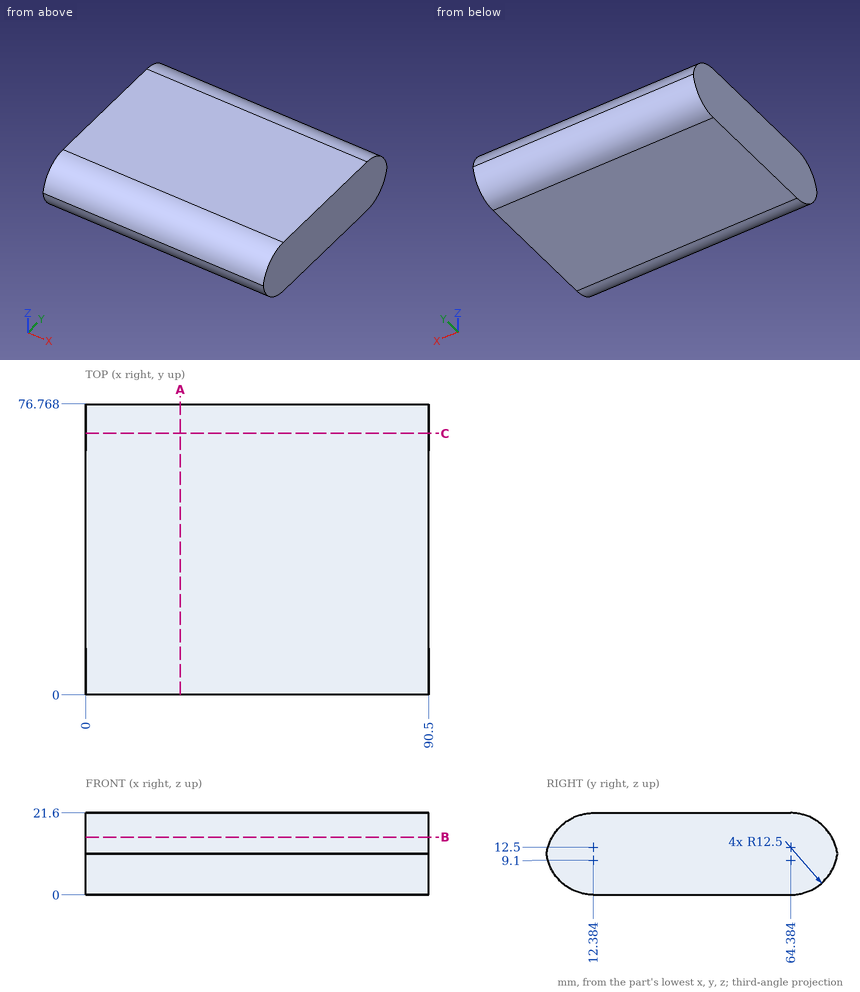
For this review, use the dimensioned drawing (mm, ordinates from the lowest corner) and the shaded views. Give positions to 0.01 mm unless a question says otherwise; leave off trailing zeros. Order: outer loops, then holes, each group sorted by start corner. A loop starts at its lowest first (then second) coordinate and runs counter-clockwise, first axis right, second up.
1) Take a section at C-C (y = 69). Give the boundary of the cut face in (x, z), then the cut area to 4 significant figures.
2) Take a section at A-A (x = 25). Give the boundary of the cut face in (y, z).
3) Wall thickness on line 1 (Z direction, x = 9, y = 65) (1 decimal); line 2 (Z direction, x = 36, y = 6); line 3 (Y direction, x = 17, z = 20) (1 decimal): over which ranges is each line inside the solid? List them lowest first.
4) Insertion check: pin 1 (8 mm diameter, centred on x = 13.5, z = 4.5, fed in from -Y). The pin has a flat end and moves straight along its axis. Give the tip position at first contact, or say it passes through.
5) Take a section at B-B (z = 15.25). Give the boundary of the cut face in (x, y).
Derived:
1. outline: (0, 0.88) - (90.5, 0.88) - (90.5, 20.72) - (0, 20.72) - close
1. area: 1,795 mm2
2. outline: (0, 10.8) arc R12.5 ccw to (12.38, 0) - (64.38, 0) arc R12.5 ccw to (76.77, 10.8) arc R12.5 ccw to (64.38, 21.6) - (12.38, 21.6) arc R12.5 ccw to start
3. line 1: z = 0 to 21.6
3. line 2: z = 1.75 to 19.85
3. line 3: y = 6.3 to 70.5
4. pin 1: stops at y = 0.54
5. outline: (0, 1.5) - (90.5, 1.5) - (90.5, 75.27) - (0, 75.27) - close
